Design review of the part built by this model. Coordinates are the model's own, in mm. A direction names the side the tool comes from. Coordinates: 2 decimals unless noted, no trailing zeros. Loops run counter-clockwise (first coordinate to the right, second up) from the corner with the lowest first, then second, coordinate; pieces in that order, holes last.
Q1. Add section B-B on x = -15.5. Give the boundary of the cut face in (y, z), and give its area (3 significant figures).
Q2. Add section C-C on y = 2.5. Give the boundary of the cut face in (x, z), and give its area (3 significant figures).
Q3. Add section D-D on z = 3. Give the boundary of the cut face in (x, y).
Q4. Wall thickness on probe 1 along X at (y, z) = (2.5, -1.75); probe 2 along Z at (x, y) = (-19, 4.25); probe 3 along X at (y, z) = (12, -5): over which ranges is each line inside the solid? List them lowest first.
Q5. Machinability: for faces 5 (the face through (-6, 5, 4.853)), 6 (the face through (15.724, 5, -3)), 7 (the face through (-28.076, 5, -3)), 8 (the face through (-6, 5, -10.147)), which of the approach directions +Z, -Z, +X, -X, +Y, -Y give a long, thin tool a straight path to every point of the face, cutting with its end or side? Answer none if there is none.
Q6. For P1, Ø2, axis at x = -10, y = 7, coming from the -Z side; P2, Ø3, axis at y = 7.5, z = 0, coming from the -X side; P3, Ø10, axis at x = -2, z = -3.5, coming from the -Y side, all flat-tipped, find the tip position at first contact; note any pin that passes through.
Q7. Add section A-A on z = -1. Give the boundary of the cut face in (x, y), and give its area (3 significant figures).
Q8. Draft analysis for pull direction Z (two halves, no side actions). For faces 1 (the face through (16.924, 5, -3)), 2 (the face through (-6, 11, -7.747)), 3 (the face through (-6, 12, -10.147)), 4 (the face through (-6, 11, -11.347)), state which applies: released by +Z, released by -Z, zero draft, split by the parting line, or undercut.
```python
from build123d import *

# Parameters (mm, degrees)
SKETCH2_W           = 45
SKETCH2_H           = 15
SKETCH2_W_2         = 42.6
SKETCH2_H_2         = 12.6
EXTRUDE_THIN1_DEPTH = 10
SKETCH5_W           = 47.4
SKETCH5_H           = 17.4
SKETCH5_W_2         = 40.2
SKETCH5_H_2         = 10.2
EXTRUDE_THIN3_DEPTH = 3
SKETCH6_W           = 45
SKETCH6_H           = 15
CUT_EXTRUDE2_DEPTH  = 1.5


with BuildPart() as part:
    # Sketch2 → Extrude-Thin1 (new body)
    with BuildSketch(Plane(origin=(0, 0, 0), x_dir=(1, 0, 0), z_dir=(0, 1, 0))):
        with Locations((-5.576315789, 2.647368421)):
            Rectangle(SKETCH2_W, SKETCH2_H)
        with Locations((-5.576315789, 2.647368421)):
            Rectangle(SKETCH2_W_2, SKETCH2_H_2, mode=Mode.SUBTRACT)
    extrude(amount=EXTRUDE_THIN1_DEPTH)

    # Sketch5 → Extrude-Thin3 (add)
    with BuildSketch(Plane(origin=(0, 10, 0), x_dir=(1, 0, 0), z_dir=(0, 1, 0))):
        with Locations((-5.576315789, 2.647368421)):
            Rectangle(SKETCH5_W, SKETCH5_H)
        with Locations((-5.576315789, 2.647368421)):
            Rectangle(SKETCH5_W_2, SKETCH5_H_2, mode=Mode.SUBTRACT)
    extrude(amount=EXTRUDE_THIN3_DEPTH)

    # Sketch6 → Cut-Extrude2 (cut)
    with BuildSketch(Plane(origin=(0, 13, 0), x_dir=(1, 0, 0), z_dir=(0, 1, 0))):
        with Locations((-5.576315789, 2.647368421)):
            Rectangle(SKETCH6_W, SKETCH6_H)
    extrude(amount=-CUT_EXTRUDE2_DEPTH, mode=Mode.SUBTRACT)


solid = part.part
```
Entries:
1. outline: (0, -10.15) - (10, -10.15) - (10, -11.35) - (13, -11.35) - (13, -10.15) - (11.5, -10.15) - (11.5, -7.75) - (10, -7.75) - (10, -8.95) - (0, -8.95) - close; (0, 3.65) - (10, 3.65) - (10, 2.45) - (11.5, 2.45) - (11.5, 4.85) - (13, 4.85) - (13, 6.05) - (10, 6.05) - (10, 4.85) - (0, 4.85) - close
1. area: 38.4 mm2
2. outline: (-28.08, -10.15) - (16.92, -10.15) - (16.92, 4.85) - (-28.08, 4.85) - close; hole (-26.88, -8.95) - (15.72, -8.95) - (15.72, 3.65) - (-26.88, 3.65) - close
2. area: 138 mm2
3. outline: (-29.28, 10) - (-28.08, 10) - (-28.08, 0) - (-26.88, 0) - (-26.88, 10) - (15.72, 10) - (15.72, 0) - (16.92, 0) - (16.92, 10) - (18.12, 10) - (18.12, 13) - (16.92, 13) - (16.92, 11.5) - (-28.08, 11.5) - (-28.08, 13) - (-29.28, 13) - close
4. probe 1: x = -28.08 to -26.88, 15.72 to 16.92
4. probe 2: z = -10.15 to -8.95, 3.65 to 4.85
4. probe 3: x = -29.28 to -28.08, 16.92 to 18.12
5. face 5: +Z, +X, -X, -Y
5. face 6: -Y
5. face 7: +Z, -Z, -X, -Y
5. face 8: -Z, +X, -X, -Y
6. P1: stops at z = -10.15
6. P2: stops at x = -28.08
6. P3: stops at y = 10
7. outline: (-29.28, 10) - (-28.08, 10) - (-28.08, 0) - (-26.88, 0) - (-26.88, 10) - (-25.68, 10) - (-25.68, 11.5) - (-28.08, 11.5) - (-28.08, 13) - (-29.28, 13) - close; (14.52, 10) - (15.72, 10) - (15.72, 0) - (16.92, 0) - (16.92, 10) - (18.12, 10) - (18.12, 13) - (16.92, 13) - (16.92, 11.5) - (14.52, 11.5) - close
7. area: 38.4 mm2
8. face 1: zero draft
8. face 2: undercut
8. face 3: undercut
8. face 4: released by -Z
